The model under review builds one solid part; all positions refer to its coordinate system, in mm. Face numbers are marked on the shaded views. Give positions to 0.01 mm unless a question says otherwise; leave off trailing zeros. Order: outer loops, then holes, each group sorted by start corner. A loop starts at its lowest first (then second) coordinate and runs counter-clockwise, first axis right, second up.
```python
from build123d import *

# Parameters (mm, degrees)
SKETCH_1_R               = 9
SKETCH_1_R_2             = 5
EXTRUDE_1_DEPTH          = 35
SKETCH_2_R               = 10
SKETCH_2_R_2             = 5
EXTRUDE_2_DEPTH          = 6
SKETCH_3_W               = 23.145336851
SKETCH_3_H               = 3
CUT_EXTRUDE_1_DEPTH      = 1
CUT_EXTRUDE_2_REACH      = 45.37
CUT_EXTRUDE_2_END_RADIUS = 10
SKETCH_4_R               = 1.5


with BuildPart() as part:
    # Эскиз1 → Бобышка-Вытянуть1 (new body)
    with BuildSketch(Plane.XY):
        Circle(SKETCH_1_R)
        Circle(SKETCH_1_R_2, mode=Mode.SUBTRACT)
    extrude(amount=EXTRUDE_1_DEPTH)

    # Эскиз2 → Бобышка-Вытянуть2 (add)
    with BuildSketch(Plane.XY.offset(35)):
        Circle(SKETCH_2_R)
        Circle(SKETCH_2_R_2, mode=Mode.SUBTRACT)
    extrude(amount=EXTRUDE_2_DEPTH)

    # Эскиз3 → Вырез-Вытянуть1 (cut)
    with BuildSketch(Plane.XY.offset(41)):
        with Locations((0.097661358, 4.999046135)):
            Rectangle(SKETCH_3_W, SKETCH_3_H)
    extrude(amount=-CUT_EXTRUDE_1_DEPTH, mode=Mode.SUBTRACT)

    # Вырез-Вытянуть2: up to this cylinder (the profile starts inside it)
    cut_extrude_2_end = Plane(origin=(0, 0, 38), z_dir=(0, 0, -1)) * Cylinder(CUT_EXTRUDE_2_END_RADIUS, 111.74, mode=Mode.PRIVATE)
    # Эскиз4 → Вырез-Вытянуть2 (cut, up to the surface)
    with BuildSketch(Plane(origin=(0, 0, 0), x_dir=(1, 0, 0), z_dir=(0, 1, 0)), mode=Mode.PRIVATE) as cut_extrude_2_sk1:
        with Locations(Location((0, -38, 0), (0, 0, 270))):
            Circle(SKETCH_4_R)
    cut_extrude_2_tool1 = extrude(cut_extrude_2_sk1.sketch, amount=-CUT_EXTRUDE_2_REACH, mode=Mode.PRIVATE) & cut_extrude_2_end
    add(cut_extrude_2_tool1.solids().sort_by_distance((0, 0, 38))[0], mode=Mode.SUBTRACT)


solid = part.part
```
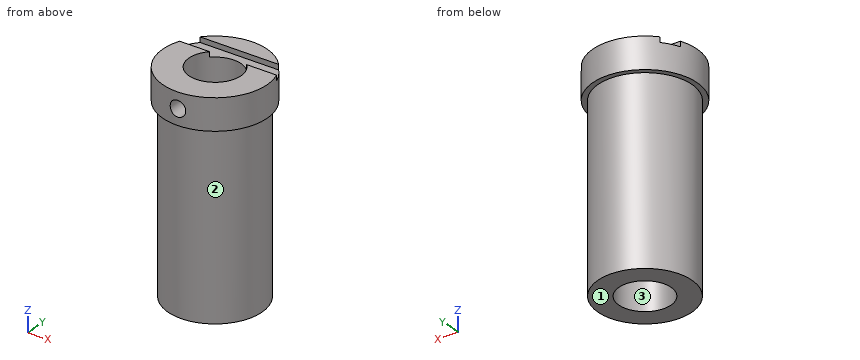
1. Insertion check: pin 1 (10 mm diameter, centred on x = -4, z = 20, fed in from +Y); pin 2 (1.1 mm diameter, centred on x = -1.5, z = 40.5, fed in from -Y); pin 3 (4 mm diameter, centred on x = 1.5, z = 5, fed in from -Y). Each pin has a flat end and moves straight along its axis. Give the tip position at first contact, or say it passes through.
2. To check wall thickness, follow line 1 (Y direction, x = 0, z = 20); line 2 (Z direction, x = 0, y = -6.45); line 3 (X direction, y = 2, z = 14). State the ranges of each line that lie inside material, in increasing order.
3. Draft analysis for pull direction Y (two halves, no side actions). For the marked faces 1, 2 and 3, state which applies: pulls with the +Y half, pulls with the -Y half, needs draft (parallel to the pull), parting line crosses it, or undercut.
4. Take a section at A-A (y = 0). Write out the cut boundary in (x, z), and give its area (3 significant figures).
5. Take a section at C-C (z = 10). Write out the cut boundary in (x, y), and give its area (3 significant figures).
6. Take a section at D-D (x = -2.5). Write out the cut boundary in (y, z).
7. Take a section at B-B (x = 0). Write out the cut boundary in (y, z), and give its area (4 significant figures).
Answer:
1. pin 1: stops at y = 9
1. pin 2: stops at y = -9.95
1. pin 3: stops at y = -9
2. line 1: y = -9 to -5, 5 to 9
2. line 2: z = 0 to 36.5, 39.5 to 41
2. line 3: x = -8.77 to -4.58, 4.58 to 8.77
3. face 1: needs draft
3. face 2: parting line crosses it
3. face 3: undercut
4. outline: (-10, 35) - (-9, 35) - (-9, 0) - (-5, 0) - (-5, 41) - (-10, 41) - close; (5, 0) - (9, 0) - (9, 35) - (10, 35) - (10, 41) - (5, 41) - close
4. area: 340 mm2
5. outline: circle Ø18 at (0, 0); hole circle Ø10 at (0, 0)
5. area: 176 mm2
6. outline: (-9.68, 35) - (-8.65, 35) - (-8.65, 0) - (-4.33, 0) - (-4.33, 41) - (-9.68, 41) - close; (4.33, 0) - (8.65, 0) - (8.65, 35) - (9.68, 35) - (9.68, 41) - (6.5, 41) - (6.5, 40) - (4.33, 40) - close
7. outline: (-10, 35) - (-9, 35) - (-9, 0) - (-5, 0) - (-5, 36.5) - (-10, 36.5) - close; (-10, 39.5) - (-5, 39.5) - (-5, 41) - (-10, 41) - close; (5, 0) - (9, 0) - (9, 35) - (10, 35) - (10, 41) - (6.5, 41) - (6.5, 40) - (5, 40) - close
7. area: 323.5 mm2
